Input: part model. Units: mm. Frame: model coordinates. A direction names the side the tool comes from. Round coordinates to 2 decimals unless told otherwise and drop trailing zeros. Order: outer loops, then holes, each group sorted by start corner. A loop starts at its lowest first (then second) coordinate and runs counter-clockwise, first axis right, second up. Notation, with made-up numbers: (-21.5, 10.5) -> (21.5, 10.5) arc R20 ccw to (21.5, 37.5) -> close; hole circle Ø9 at (-25, 47.5). An arc over 180 degrees is marked (long way). Use a Markdown table: item, result.
from build123d import *

# Parameters (mm, degrees)
SKETCH_1_R          = 3
EXTRUDE_1_DEPTH     = 5
EXTRUDE_3_DEPTH     = 10
EXTRUDE_4_DEPTH     = 15
EXTRUDE_5_DEPTH     = 4
CUT_EXTRUDE_1_DEPTH = 3.5


with BuildPart() as part:
    # 草图1 → 凸台-拉伸1 (new body)
    with BuildSketch(Plane.XY):
        with BuildLine():
            Line((-15, 10), (15, 10))
            ThreePointArc((15, 10), (25, 0), (15, -10))
            Line((15, -10), (-15, -10))
            ThreePointArc((-15, -10), (-25, 0), (-15, 10))
        make_face()
        with Locations((-15, 0)):
            Circle(SKETCH_1_R, mode=Mode.SUBTRACT)
        with Locations((15, 0)):
            Circle(SKETCH_1_R, mode=Mode.SUBTRACT)
    extrude(amount=EXTRUDE_1_DEPTH)

    # 草图4 → 凸台-拉伸3 (add)
    with BuildSketch(Plane.XY):
        with BuildLine():
            Line((7.062746067, 0), (-7.062746067, 0))
            ThreePointArc((-7.062746067, 0), (-7.724183895, -0.25), (-8.054902808, -0.875))
            ThreePointArc((-8.054902808, -0.875), (-10.197413633, -5.092657871), (-14.533333333, -6.984427122))
            ThreePointArc((-14.533333333, -6.984427122), (-14.865148372, -7.141749748), (-15, -7.483314774))
            Line((-15, -7.483314774), (-15, -9.5))
            ThreePointArc((-15, -9.5), (-14.853553391, -9.853553391), (-14.5, -10))
            Line((-14.5, -10), (14.5, -10))
            ThreePointArc((14.5, -10), (14.853553391, -9.853553391), (15, -9.5))
            Line((15, -9.5), (15, -7.483314774))
            ThreePointArc((15, -7.483314774), (14.865148372, -7.141749748), (14.533333333, -6.984427122))
            ThreePointArc((14.533333333, -6.984427122), (10.197413633, -5.092657871), (8.054902808, -0.875))
            ThreePointArc((8.054902808, -0.875), (7.724183895, -0.25), (7.062746067, 0))
        make_face()
    extrude(amount=EXTRUDE_3_DEPTH)

    # 草图5 → 凸台-拉伸4 (add)
    with BuildSketch(Plane.XY.offset(10)):
        with BuildLine():
            Line((-15, -7.483314774), (-15, -9.5))
            ThreePointArc((-15, -9.5), (-14.853553391, -9.853553391), (-14.5, -10))
            Line((-14.5, -10), (14.5, -10))
            ThreePointArc((14.5, -10), (14.853553391, -9.853553391), (15, -9.5))
            Line((15, -9.5), (15, -7.483314774))
            ThreePointArc((15, -7.483314774), (14.853553391, -7.129761383), (14.5, -6.983314774))
            Line((14.5, -6.983314774), (-14.5, -6.983314774))
            ThreePointArc((-14.5, -6.983314774), (-14.853553391, -7.129761383), (-15, -7.483314774))
        make_face()
    extrude(amount=EXTRUDE_4_DEPTH)

    # 草图9 → 凸台-拉伸5 (add, symmetric)
    with BuildSketch(Plane(origin=(0, 0, 0), x_dir=(0, 0, -1), z_dir=(1, 0, 0))):
        Polygon((-25, -6.983314774), (-10, -6.983314774), (-10, -1.983314774), align=None)
    extrude(amount=EXTRUDE_5_DEPTH, both=True)

    # 草图10 → 切除-拉伸1 (cut)
    with BuildSketch(Plane(origin=(0, -6.983314774, 0), x_dir=(1, 0, 0), z_dir=(0, 1, 0))):
        with BuildLine():
            Line((10, -13.525), (8, -13.525))
            ThreePointArc((8, -13.525), (6.525, -15), (8, -16.475))
            Line((8, -16.475), (10, -16.475))
            ThreePointArc((10, -16.475), (11.475, -15), (10, -13.525))
        make_face()
        with BuildLine():
            Line((8, -19.525), (10, -19.525))
            ThreePointArc((10, -19.525), (11.475, -21), (10, -22.475))
            Line((10, -22.475), (8, -22.475))
            ThreePointArc((8, -22.475), (6.525, -21), (8, -19.525))
        make_face()
        with BuildLine():
            Line((-10, -13.525), (-8, -13.525))
            ThreePointArc((-8, -13.525), (-6.525, -15), (-8, -16.475))
            Line((-8, -16.475), (-10, -16.475))
            ThreePointArc((-10, -16.475), (-11.475, -15), (-10, -13.525))
        make_face()
        with BuildLine():
            Line((-8, -19.525), (-10, -19.525))
            ThreePointArc((-10, -19.525), (-11.475, -21), (-10, -22.475))
            Line((-10, -22.475), (-8, -22.475))
            ThreePointArc((-8, -22.475), (-6.525, -21), (-8, -19.525))
        make_face()
    extrude(amount=-CUT_EXTRUDE_1_DEPTH, mode=Mode.SUBTRACT)


solid = part.part
1) Ray query, probe 1 along Y at (x, z) = (-15, 1.3); probe 2 along X at (y, z) = (-4, 12.5); probe 3 along Z at (x, y) = (-10, -5). Return the intervals inside material, ascending.
Answer key:
| item | result |
|---|---|
| probe 1 | y = -10 to -3, 3 to 10 |
| probe 2 | x = -4 to 4 |
| probe 3 | z = 0 to 10 |
2) Cut plane A-A on x = -1.5. Return loops of the section in (y, z).
Answer key:
| item | result |
|---|---|
| outline | (-10, 0) -> (10, 0) -> (10, 5) -> (0, 5) -> (0, 10) -> (-1.98, 10) -> (-6.98, 25) -> (-10, 25) -> close |
3) Cut plane C-C on y = -8.5. Return loops of the section in (x, z) (3 decimals), and give its area (3 significant figures).
Answer key:
| item | result |
|---|---|
| outline | (-20.268, 0) -> (20.268, 0) -> (20.268, 5) -> (15, 5) -> (15, 25) -> (-15, 25) -> (-15, 5) -> (-20.268, 5) -> close; hole (-10, 13.525) -> (-8, 13.525) arc R1.475 ccw to (-8, 16.475) -> (-10, 16.475) arc R1.475 ccw to start; hole (-10, 19.525) -> (-8, 19.525) arc R1.475 ccw to (-8, 22.475) -> (-10, 22.475) arc R1.475 ccw to start; hole (8, 13.525) -> (10, 13.525) arc R1.475 ccw to (10, 16.475) -> (8, 16.475) arc R1.475 ccw to start; hole (8, 19.525) -> (10, 19.525) arc R1.475 ccw to (10, 22.475) -> (8, 22.475) arc R1.475 ccw to start |
| area | 752 mm^2 |
4) Contact query for flat-ended pins moving along their axis: P1, Ø1.6, axis at y = -8, z = 13.5, coming from the -X side; P2, Ø2.5, axis at x = 2, z = 8.5, coming from the +Y side; P3, Ø4, axis at y = -3.5, z = 19.5, coming from the -X side. Output: stop coordinate, or through.
Answer key:
| item | result |
|---|---|
| P1 | stops at x = -15 |
| P2 | stops at y = 0 |
| P3 | stops at x = -4 |
5) Cut plane D-D on z = 4.25. Return loops of the section in (x, y).
Answer key:
| item | result |
|---|---|
| outline | (-15, -10) -> (15, -10) arc R10 ccw to (15, 10) -> (-15, 10) arc R10 ccw to start; hole circle Ø6 at (-15, 0); hole circle Ø6 at (15, 0) |
6) Draft query along Z for faces 1 (the face through (0, 2, 5)), 2 (the face through (0, -10, 12)), 3 (the face through (-6.525, -8.471, 14.968)). Return one class per face: released by +Z, released by -Z, zero draft, split by the parting line, or undercut.
Answer key:
| item | result |
|---|---|
| face 1 | released by +Z |
| face 2 | zero draft |
| face 3 | undercut |
7) Set-up query: faces 4 (the face through (15, -9, 15)), 5 (the face through (4, -6, 14)), 6 (the face through (0, -1, 10)), 7 (the face through (-9, -8, 22.475)). Return all of +Z, -Z, +X, -X, +Y, -Y with unobstructed straight access to the full face (end or side cutting, diameter ignored); none if empty.
Answer key:
| item | result |
|---|---|
| face 4 | +Z, +X, +Y, -Y |
| face 5 | +Z, +X, +Y |
| face 6 | +Z, +Y |
| face 7 | +Y, -Y |
8) Cut plane B-B on z = 14.75. Return loops of the section in (x, y), and give its area (3 significant figures).
Answer key:
| item | result |
|---|---|
| outline | (-15, -9.5) arc R0.5 ccw to (-14.5, -10) -> (-11.45, -10) -> (-11.45, -6.98) -> (-14.5, -6.98) arc R0.5 ccw to (-15, -7.48) -> close; (-6.55, -10) -> (6.55, -10) -> (6.55, -6.98) -> (4, -6.98) -> (4, -3.57) -> (-4, -3.57) -> (-4, -6.98) -> (-6.55, -6.98) -> close; (11.45, -10) -> (14.5, -10) arc R0.5 ccw to (15, -9.5) -> (15, -7.48) arc R0.5 ccw to (14.5, -6.98) -> (11.45, -6.98) -> close |
| area | 88.0 mm^2 |
